from build123d import *

# Parameters (mm, degrees)
F2_DEPTH = 25.4
F3_W     = 14.732
F3_H     = 0.635
F4_DEPTH = 3.81
F6_DEPTH = 3.81
F7_D     = 3.81


# Not quite as in the source:
# - a feature of the source that left no trace in its solid (it failed there, or was rolled back) is left out
# - a feature names something its author has since deleted; it is built from what else it names


with BuildPart() as f2:
    # F1 (on Front) → F2 (new body)
    with BuildSketch(Plane.XZ):
        with BuildLine():
            Line((-4.826, 5.08), (4.826, 5.08))
            ThreePointArc((4.826, 5.08), (5.7240256121, 4.7080256121), (6.096, 3.81))
            Line((6.096, 3.81), (6.096, -5.08))
            Line((6.096, -5.08), (16.256, -5.08))
            Line((16.256, -5.08), (16.256, -2.54))
            Line((16.256, -2.54), (8.636, -2.54))
            Line((8.636, -2.54), (8.636, 6.35))
            ThreePointArc((8.636, 6.35), (8.2640256121, 7.2480256121), (7.366, 7.62))
            Line((7.366, 7.62), (-7.366, 7.62))
            ThreePointArc((-7.366, 7.62), (-8.2640256121, 7.2480256121), (-8.636, 6.35))
            Line((-8.636, 6.35), (-8.636, -2.54))
            Line((-8.636, -2.54), (-16.256, -2.54))
            Line((-16.256, -2.54), (-16.256, -5.08))
            Line((-16.256, -5.08), (-6.096, -5.08))
            Line((-6.096, -5.08), (-6.096, 3.81))
            ThreePointArc((-6.096, 3.81), (-5.7240256121, 4.7080256121), (-4.826, 5.08))
        make_face()
    extrude(amount=F2_DEPTH)

    # F3 (on face) → F4 (join)
    with BuildSketch(Plane.XY.offset(7.62)):
        with Locations((0, -0.3175)):
            Rectangle(F3_W, F3_H)
    extrude(amount=-F4_DEPTH)

    # F3 (on face) → F6 (join)
    with BuildSketch(Plane.XY.offset(7.62)):
        with Locations((0, -25.0825)):
            Rectangle(F3_W, F3_H)
    extrude(amount=-F6_DEPTH)

    # F7 (through all)
    with Locations(Plane.XY.offset(-2.54)):
        with Locations((-12.446, -12.7), (12.446, -12.7)):
            Hole(F7_D / 2)


solid = f2.part
Here's how the part is built. I have some questions about the finished solid (model axes, mm). A direction names the side the tool comes from. Round coordinates to 2 decimals unless told otherwise and drop trailing zeros. Order: outer loops, then holes, each group sorted by start corner. A loop starts at its lowest first (then second) coordinate and runs counter-clockwise, first axis right, second up. Notation, with made-up numbers: (70, 60.5) -> (90, 60.5) arc R12 ccw to (90, 68.5) -> close; hole circle Ø2 at (16, 27). An arc over 180 degrees is marked (long way). Return JSON: item names as keys, results as strings.
Q1. If we section it at A-A on y = -12.7: List the corners of the cut face in (x, z) for me, plus the area to 3 significant figures.
Filled sheet:
{"outline": "(-16.26, -5.08) -> (-14.35, -5.08) -> (-14.35, -2.54) -> (-16.26, -2.54) -> close; (-10.54, -5.08) -> (-6.1, -5.08) -> (-6.1, 3.81) arc R1.27 cw to (-4.83, 5.08) -> (4.83, 5.08) arc R1.27 cw to (6.1, 3.81) -> (6.1, -5.08) -> (10.54, -5.08) -> (10.54, -2.54) -> (8.64, -2.54) -> (8.64, 6.35) arc R1.27 ccw to (7.37, 7.62) -> (-7.37, 7.62) arc R1.27 ccw to (-8.64, 6.35) -> (-8.64, -2.54) -> (-10.54, -2.54) -> close; (14.35, -5.08) -> (16.26, -5.08) -> (16.26, -2.54) -> (14.35, -2.54) -> close", "area": "115 mm^2"}
Q2. If we mould it in two halves opening along Y, with no side actions, what happens to faces 6 (the flat face through (0, -13, 5.08)), 7 (the flat face through (15, -13, -2.54)), 8 (the flat face through (0, 0, 4))? For each: released by +Y, released by -Y, zero draft, split by the parting line, or undercut.
Filled sheet:
{"face 6": "undercut", "face 7": "zero draft", "face 8": "released by +Y"}
Q3. I need wall thicknesses on line 1 along X through (y, z) = (-24, 2.75); line 2 along X through (y, z) = (-22.25, -4); line 3 along Z through (x, y) = (-3, -1.75). Which ranges of each line are inside material? Lowest first, please. Write a range as from..to.
Filled sheet:
{"line 1": "x = -8.64..-6.1, 6.1..8.64", "line 2": "x = -16.26..-6.1, 6.1..16.26", "line 3": "z = 5.08..7.62"}
Q4. Which directions (+Z, -Z, +X, -X, +Y, -Y) give clear straight access to the entire face, cutting with the end or side of a thin tool? Please do faces 1 (the flat face through (6.096, -13, -1)), 2 (the flat face through (-8.636, -13, 2)), 3 (the cylindrical face through (-5.73, -12.53, 4.7)), 4 (the flat face through (10, -13, -5.08)), 5 (the flat face through (8.636, -13, 2)).
Filled sheet:
{"face 1": "-Z, +Y, -Y", "face 2": "+Z, -X, +Y, -Y", "face 3": "-Z", "face 4": "-Z, +X, -X, +Y, -Y", "face 5": "+Z, +X, +Y, -Y"}
Q5. If we section it at D-D on y = -18.5: List the corners of the cut face in (x, z) for me, plus the area to 3 significant figures.
Filled sheet:
{"outline": "(-16.26, -5.08) -> (-6.1, -5.08) -> (-6.1, 3.81) arc R1.27 cw to (-4.83, 5.08) -> (4.83, 5.08) arc R1.27 cw to (6.1, 3.81) -> (6.1, -5.08) -> (16.26, -5.08) -> (16.26, -2.54) -> (8.64, -2.54) -> (8.64, 6.35) arc R1.27 ccw to (7.37, 7.62) -> (-7.37, 7.62) arc R1.27 ccw to (-8.64, 6.35) -> (-8.64, -2.54) -> (-16.26, -2.54) -> close", "area": "134 mm^2"}
Q6. If we section it at C-C on x = 13.5: List the corners of the cut face in (y, z) for me.
Filled sheet:
{"outline": "(-25.4, -5.08) -> (-14.29, -5.08) -> (-14.29, -2.54) -> (-25.4, -2.54) -> close; (-11.11, -5.08) -> (0, -5.08) -> (0, -2.54) -> (-11.11, -2.54) -> close"}
Q7. If we section it at B-B on z = 2.75: List the corners of the cut face in (x, y) for me.
Filled sheet:
{"outline": "(-8.64, -25.4) -> (-6.1, -25.4) -> (-6.1, 0) -> (-8.64, 0) -> close; (6.1, -25.4) -> (8.64, -25.4) -> (8.64, 0) -> (6.1, 0) -> close"}
Q8. For pin 1 Ø4 at (x, y) = (13.5, -16.5) entering from +Z; pin 2 Ø3.5 at (x, y) = (-12.446, -12.7) entering from -Z; pin 3 Ø4 at (y, z) = (-8.5, 3.5) entering from +X; pin 4 Ø0.7 at (x, y) = (2.5, -25) entering from -Z, each with a flat end and sliding along its axis, tell me the tip position at first contact or that it passes through.
Filled sheet:
{"pin 1": "stops at z = -2.54", "pin 2": "passes through", "pin 3": "stops at x = 8.64", "pin 4": "stops at z = 3.81"}
